Read the model definition and answer for the solid it produces. Units are mm, in the model's axes. Give positions to 0.01 mm unless a question says otherwise; leave off trailing zeros. Write each loop counter-clockwise with the first axis right and the second up, starting at its lowest first coordinate (ties: lowest second). Pieces come first, ordered by that corner, then holes. Notation, with made-up numbers: (-8.5, 17.25) - (44.5, 17.25) arc R22 ccw to (44.5, 49.25) - close; hole circle Ø10 at (56.25, -3). An arc over 180 degrees is marked (long way). Answer as a JSON object with one key per item and string values. Group by question number.
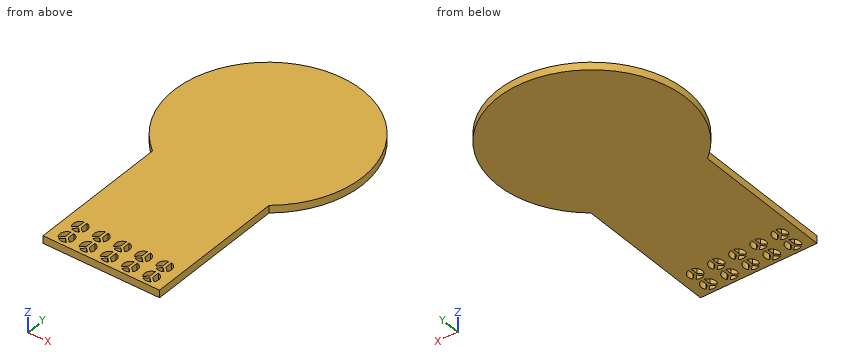
```python
from build123d import *

# Parameters (mm, degrees)
EXTRUDE_1_DEPTH     = 8
CUT_EXTRUDE_1_DEPTH = 10


with BuildPart() as part:
    # 草图1 → 凸台-拉伸1 (new body)
    with BuildSketch(Plane.XY):
        with BuildLine():
            Line((0, 0), (124, 0))
            Line((124, 0), (124, 150))
            ThreePointArc((124, 150), (62, 328.460180984), (0, 150))
            Line((0, 150), (0, 0))
        make_face()
    extrude(amount=EXTRUDE_1_DEPTH)

    # 草图2 → 切除-拉伸1 (cut)
    with BuildSketch(Plane.XY.offset(8)):
        with BuildLine():
            Line((38.000879916, 18.335012989), (38.000879916, 10.614550667))
            Line((38.000879916, 10.614550667), (33.500377126, 6.485861413))
            ThreePointArc((33.500377126, 6.485861413), (32.48869593, 13.649372886), (38.000879916, 18.335012989))
        make_face()
        with BuildLine():
            Line((40.999120084, 18.335012989), (40.999120084, 10.614550667))
            Line((40.999120084, 10.614550667), (45.499622874, 6.485861413))
            ThreePointArc((45.499622874, 6.485861413), (46.51130407, 13.649372886), (40.999120084, 18.335012989))
        make_face()
        with BuildLine():
            Line((43.629589922, 4.725654413), (39.494098953, 8.861145382))
            Line((39.494098953, 8.861145382), (35.363302178, 4.730348608))
            ThreePointArc((35.363302178, 4.730348608), (39.495740959, 3.486365412), (43.629589922, 4.725654413))
        make_face()
        with BuildLine():
            Line((60.500879916, 18.335012989), (60.500879916, 10.614550667))
            Line((60.500879916, 10.614550667), (56.000377126, 6.485861413))
            ThreePointArc((56.000377126, 6.485861413), (54.98869593, 13.649372886), (60.500879916, 18.335012989))
        make_face()
        with BuildLine():
            Line((63.499120084, 18.335012989), (63.499120084, 10.614550667))
            Line((63.499120084, 10.614550667), (67.999622874, 6.485861413))
            ThreePointArc((67.999622874, 6.485861413), (69.01130407, 13.649372886), (63.499120084, 18.335012989))
        make_face()
        with BuildLine():
            Line((66.129589922, 4.725654413), (61.994098953, 8.861145382))
            Line((61.994098953, 8.861145382), (57.863302178, 4.730348608))
            ThreePointArc((57.863302178, 4.730348608), (61.995740959, 3.486365412), (66.129589922, 4.725654413))
        make_face()
        with BuildLine():
            Line((83.000879916, 18.335012989), (83.000879916, 10.614550667))
            Line((83.000879916, 10.614550667), (78.500377126, 6.485861413))
            ThreePointArc((78.500377126, 6.485861413), (77.48869593, 13.649372886), (83.000879916, 18.335012989))
        make_face()
        with BuildLine():
            Line((85.999120084, 18.335012989), (85.999120084, 10.614550667))
            Line((85.999120084, 10.614550667), (90.499622874, 6.485861413))
            ThreePointArc((90.499622874, 6.485861413), (91.51130407, 13.649372886), (85.999120084, 18.335012989))
        make_face()
        with BuildLine():
            Line((88.629589922, 4.725654413), (84.494098953, 8.861145382))
            Line((84.494098953, 8.861145382), (80.363302178, 4.730348608))
            ThreePointArc((80.363302178, 4.730348608), (84.495740959, 3.486365412), (88.629589922, 4.725654413))
        make_face()
        with BuildLine():
            Line((105.500879916, 18.335012989), (105.500879916, 10.614550667))
            Line((105.500879916, 10.614550667), (101.000377126, 6.485861413))
            ThreePointArc((101.000377126, 6.485861413), (99.98869593, 13.649372886), (105.500879916, 18.335012989))
        make_face()
        with BuildLine():
            Line((108.499120084, 18.335012989), (108.499120084, 10.614550667))
            Line((108.499120084, 10.614550667), (112.999622874, 6.485861413))
            ThreePointArc((112.999622874, 6.485861413), (114.01130407, 13.649372886), (108.499120084, 18.335012989))
        make_face()
        with BuildLine():
            Line((111.129589922, 4.725654413), (106.994098953, 8.861145382))
            Line((106.994098953, 8.861145382), (102.863302178, 4.730348608))
            ThreePointArc((102.863302178, 4.730348608), (106.995740959, 3.486365412), (111.129589922, 4.725654413))
        make_face()
        with BuildLine():
            Line((38.000879916, 36.335012989), (38.000879916, 28.614550667))
            Line((38.000879916, 28.614550667), (33.500377126, 24.485861413))
            ThreePointArc((33.500377126, 24.485861413), (32.48869593, 31.649372886), (38.000879916, 36.335012989))
        make_face()
        with BuildLine():
            Line((40.999120084, 36.335012989), (40.999120084, 28.614550667))
            Line((40.999120084, 28.614550667), (45.499622874, 24.485861413))
            ThreePointArc((45.499622874, 24.485861413), (46.51130407, 31.649372886), (40.999120084, 36.335012989))
        make_face()
        with BuildLine():
            Line((15.500879916, 18.335012989), (15.500879916, 10.614550667))
            Line((15.500879916, 10.614550667), (11.000377126, 6.485861413))
            ThreePointArc((11.000377126, 6.485861413), (9.98869593, 13.649372886), (15.500879916, 18.335012989))
        make_face()
        with BuildLine():
            Line((18.499120084, 18.335012989), (18.499120084, 10.614550667))
            Line((18.499120084, 10.614550667), (22.999622874, 6.485861413))
            ThreePointArc((22.999622874, 6.485861413), (24.01130407, 13.649372886), (18.499120084, 18.335012989))
        make_face()
        with BuildLine():
            Line((21.129589922, 4.725654413), (16.994098953, 8.861145382))
            Line((16.994098953, 8.861145382), (12.863302178, 4.730348608))
            ThreePointArc((12.863302178, 4.730348608), (16.995740959, 3.486365412), (21.129589922, 4.725654413))
        make_face()
        with BuildLine():
            Line((43.629589922, 22.725654413), (39.494098953, 26.861145382))
            Line((39.494098953, 26.861145382), (35.363302178, 22.730348608))
            ThreePointArc((35.363302178, 22.730348608), (39.495740959, 21.486365412), (43.629589922, 22.725654413))
        make_face()
        with BuildLine():
            Line((60.500879916, 36.335012989), (60.500879916, 28.614550667))
            Line((60.500879916, 28.614550667), (56.000377126, 24.485861413))
            ThreePointArc((56.000377126, 24.485861413), (54.98869593, 31.649372886), (60.500879916, 36.335012989))
        make_face()
        with BuildLine():
            Line((63.499120084, 36.335012989), (63.499120084, 28.614550667))
            Line((63.499120084, 28.614550667), (67.999622874, 24.485861413))
            ThreePointArc((67.999622874, 24.485861413), (69.01130407, 31.649372886), (63.499120084, 36.335012989))
        make_face()
        with BuildLine():
            Line((66.129589922, 22.725654413), (61.994098953, 26.861145382))
            Line((61.994098953, 26.861145382), (57.863302178, 22.730348608))
            ThreePointArc((57.863302178, 22.730348608), (61.995740959, 21.486365412), (66.129589922, 22.725654413))
        make_face()
        with BuildLine():
            Line((83.000879916, 36.335012989), (83.000879916, 28.614550667))
            Line((83.000879916, 28.614550667), (78.500377126, 24.485861413))
            ThreePointArc((78.500377126, 24.485861413), (77.48869593, 31.649372886), (83.000879916, 36.335012989))
        make_face()
        with BuildLine():
            Line((85.999120084, 36.335012989), (85.999120084, 28.614550667))
            Line((85.999120084, 28.614550667), (90.499622874, 24.485861413))
            ThreePointArc((90.499622874, 24.485861413), (91.51130407, 31.649372886), (85.999120084, 36.335012989))
        make_face()
        with BuildLine():
            Line((88.629589922, 22.725654413), (84.494098953, 26.861145382))
            Line((84.494098953, 26.861145382), (80.363302178, 22.730348608))
            ThreePointArc((80.363302178, 22.730348608), (84.495740959, 21.486365412), (88.629589922, 22.725654413))
        make_face()
        with BuildLine():
            Line((105.500879916, 36.335012989), (105.500879916, 28.614550667))
            Line((105.500879916, 28.614550667), (101.000377126, 24.485861413))
            ThreePointArc((101.000377126, 24.485861413), (99.98869593, 31.649372886), (105.500879916, 36.335012989))
        make_face()
        with BuildLine():
            Line((108.499120084, 36.335012989), (108.499120084, 28.614550667))
            Line((108.499120084, 28.614550667), (112.999622874, 24.485861413))
            ThreePointArc((112.999622874, 24.485861413), (114.01130407, 31.649372886), (108.499120084, 36.335012989))
        make_face()
        with BuildLine():
            Line((111.129589922, 22.725654413), (106.994098953, 26.861145382))
            Line((106.994098953, 26.861145382), (102.863302178, 22.730348608))
            ThreePointArc((102.863302178, 22.730348608), (106.995740959, 21.486365412), (111.129589922, 22.725654413))
        make_face()
        with BuildLine():
            Line((15.500879916, 36.335012989), (15.500879916, 28.614550667))
            Line((15.500879916, 28.614550667), (11.000377126, 24.485861413))
            ThreePointArc((11.000377126, 24.485861413), (9.98869593, 31.649372886), (15.500879916, 36.335012989))
        make_face()
        with BuildLine():
            Line((18.499120084, 36.335012989), (18.499120084, 28.614550667))
            Line((18.499120084, 28.614550667), (22.999622874, 24.485861413))
            ThreePointArc((22.999622874, 24.485861413), (24.01130407, 31.649372886), (18.499120084, 36.335012989))
        make_face()
        with BuildLine():
            Line((21.129589922, 22.725654413), (16.994098953, 26.861145382))
            Line((16.994098953, 26.861145382), (12.863302178, 22.730348608))
            ThreePointArc((12.863302178, 22.730348608), (16.995740959, 21.486365412), (21.129589922, 22.725654413))
        make_face()
    extrude(amount=-CUT_EXTRUDE_1_DEPTH, mode=Mode.SUBTRACT)


solid = part.part
```
1) Find section C-C, the plane x = -24. Write down the section's boundary in (y, z).
2) Find the intervals of material crossed by line 1 (Y direction, x = 39.5, z = 2.75); line 2 (X direction, y = 112, z = 2.25); line 3 (Y direction, x = 90, z = 1.5), in increasing order. Write a range as [from, to].
3) Find section B-B, the plane z = 6. Give the number of separate pieces and of enclosed holes in the cut face, and give its area (3 significant figures).
4) Find section A-A, the plane y = 96. Write down the section's boundary in (x, z), and give its area (3 significant figures).
5) Flat-ended cylindrical pins translate along their axes: pin 1 Ø1.5 at (y, z) = (163, 3.5) entering from -X; pin 2 Ø2.5 at (y, z) = (15, 5.5) entering from +X; pin 3 Ø3 at (y, z) = (250.5, 4) entering from -X. Find the tip coordinate at first contact, or state that the pin passes through.
Values follow:
{
 "1": {"outline": "(177.43, 0) - (279.49, 0) - (279.49, 8) - (177.43, 8) - close"},
 "2": {"line 1": "y = [0, 3.49], [8.86, 21.49], [26.86, 325.9]", "line 2": "x = [0, 124]", "line 3": "y = [0, 6.94], [16.09, 24.94], [34.09, 324.46]"},
 "3": {"separate pieces": "1", "enclosed holes": "30", "area": "47,000 mm2"},
 "4": {"outline": "(0, 0) - (124, 0) - (124, 8) - (0, 8) - close", "area": "992 mm2"},
 "5": {"pin 1": "stops at x = -14.24", "pin 2": "stops at x = 124", "pin 3": "stops at x = -35.87"}
}
